Check sheet for the drawn part. Datum: minimum x, y, z corner. Units: mm. A direction names the side the tool comes from. Coordinates: 2 decimals unless noted, no trailing zeros. Write each loop counter-clockwise with the first axis right and the second up, starting at its lowest first coordinate (ties: lowest second). Pieces come first, ordered by that corner, then holes. Notation, with made-up numbers: (-3, -36) -> (17, -36) arc R29 cw to (17, -12) -> close; hole circle Ø11 at (-40, 48.25). An arc over 180 degrees is marked (long way). Write item = value, one per line. Start each with the question number.
(1) Section check A-A (y = 15). Record the cut outline in (x, z).
(2) Section check C-C (x = 17.5). Record the cut outline in (y, z), plus the area to 3 significant figures.
(3) Mould release check, pull along Z, two halves, no side actions. Record for the marked faces 1, 2 and 3: released by +Z, released by -Z, zero draft, split by the parting line, or undercut.
(4) Section check B-B (z = 9.5). Record the cut outline in (x, y).
(5) Set-up check for the marked faces 4 and 5: record each of +Z, -Z, +X, -X, +Y, -Y from which the full face is reachable in a straight line by a thin tool's end or side.
(6) Material ranges on probe 1 along X at (y, z) = (17.5, 16); probe 2 along Z at (x, y) = (26, 3), recorded low to high. Write a range as [from, to].
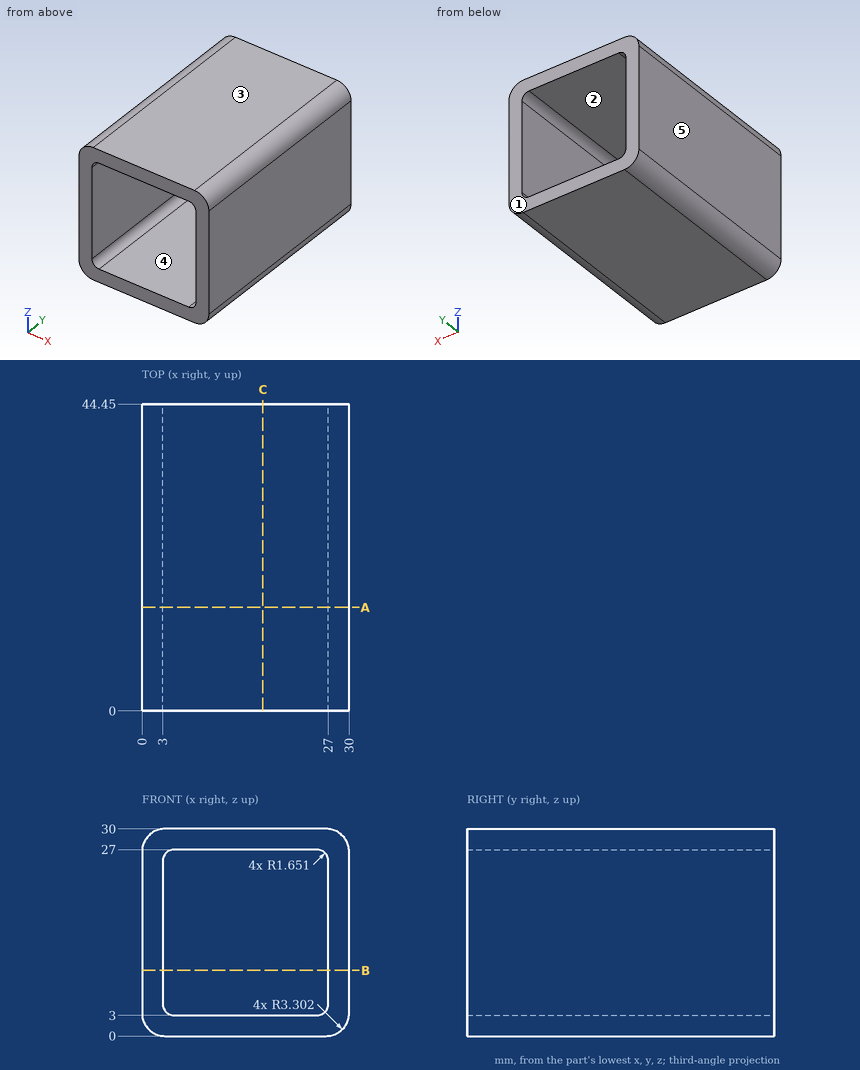
Response:
q1.outline = (0, 3.3) arc R3.3 ccw to (3.3, 0) -> (26.7, 0) arc R3.3 ccw to (30, 3.3) -> (30, 26.7) arc R3.3 ccw to (26.7, 30) -> (3.3, 30) arc R3.3 ccw to (0, 26.7) -> close; hole (3, 4.65) arc R1.65 ccw to (4.65, 3) -> (25.35, 3) arc R1.65 ccw to (27, 4.65) -> (27, 25.35) arc R1.65 ccw to (25.35, 27) -> (4.65, 27) arc R1.65 ccw to (3, 25.35) -> close
q2.outline = (0, 0) -> (44.45, 0) -> (44.45, 3) -> (0, 3) -> close; (0, 27) -> (44.45, 27) -> (44.45, 30) -> (0, 30) -> close
q2.area = 267 mm2
q3.face_1 = zero draft
q3.face_2 = undercut
q3.face_3 = released by +Z
q4.outline = (0, 0) -> (3, 0) -> (3, 44.45) -> (0, 44.45) -> close; (27, 0) -> (30, 0) -> (30, 44.45) -> (27, 44.45) -> close
q5.face_4 = +Y, -Y
q5.face_5 = +Z, -Z, -X, +Y, -Y
q6.probe_1 = [0, 3], [27, 30]
q6.probe_2 = [0, 3.13], [26.87, 30]
